Verification items for the finished model (mm, model axes). Coordinates: 2 decimals unless noted, no trailing zeros. Loops run counter-clockwise (first coordinate to the right, second up) from the corner with the lowest first, then second, coordinate; pieces in that order, holes last. Notation, with made-up numbers: (48.25, -34.5) - (84.25, -34.5) arc R20 ccw to (84.25, -26.5) - close; hole circle Ø6 at (-25.75, 26). An arc over 180 degrees is marked (long way). One line per item, written item: value. Start each with the question number.
(1) Section check D-D (x = 24). Record the boundary of the cut face in (y, z), plus the area to 3 significant figures.
(2) Section check A-A (y = 4.5). Record the boundary of the cut face in (x, z).
(3) Thickness scan on probe 1 along Y at (x, z) = (34.5, 2.35); probe 2 along Y at (x, z) = (-5, 4.2); probe 3 along X at (y, z) = (-11.5, 4.1). Record the ranges inside material, lowest first. Write a range as [from, to].
(4) Gauge pin test, flat ends, axial feed: P1, Ø3, axis at y = 7, z = 2.5, coming from the +X side; P2, Ø2, axis at y = 21.5, z = 1, coming from the +X side. Record the tip position at first contact, or that the pin passes through.
(5) Section check B-B (x = 34.5). Record the boundary of the cut face in (y, z).
(6) Section check C-C (z = 3.35). Count the separate pieces of the cut face and the enclosed holes in it, plus the area to 3 significant figures.
Autodesk Inventor part; units mm, degrees
ref_plane "YZ Plane" through (0, 0, 0) normal (1, 0, 0) x (0, 1, 0)
ref_plane "XZ Plane" through (0, 0, 0) normal (0, 1, 0) x (-1, 0, 0)
ref_plane "XY Plane" through (0, 0, 0) normal (0, 0, 1) x (1, 0, 0)
sketch "Base" plane through (0, 0, 0) normal (0, 0, 1) x (1, 0, 0)
  circle A0 centre (14.2875, 0) radius 14.2875 construction
  circle A1 centre (34.9097, 11.9062) radius 1.9939 construction
  circle A2 centre (34.9097, -11.9063) radius 1.9939 construction
  circle A3 centre (14.2875, -23.8125) radius 1.9939 construction
  circle A4 centre (-6.3347, -11.9062) radius 1.9939 construction
  circle A5 centre (-6.3347, 11.9063) radius 1.9939 construction
  circle A6 centre (14.2875, 23.8125) radius 1.9939 construction
  circle A7 centre (14.2875, 0) radius 27.5127
  arc A8 (34.1709, -15.825) -> (37.934, -9.307) centre (34.9097, -11.9063) ccw construction
  circle A9 centre (-6.3347, 11.9063) radius 1.7272
  circle A10 centre (14.2875, 23.8125) radius 1.7272
  circle A11 centre (34.9097, 11.9062) radius 1.7272
  circle A12 centre (34.9097, -11.9063) radius 1.7272
  circle A13 centre (14.2875, -23.8125) radius 1.7272
  circle A14 centre (-6.3347, -11.9062) radius 1.7272
  point P0 (0, 0)
  dimension "d3" = 55.0254
  dimension "d10" = 3.4544
extrude "Plate1" add sketch "Base" along normal blind 5
sketch "WheelMagnetAlignmentFlangeMountHoles" plane through (14.2875, 0, 0) normal (0, 0, -1) x (-1, 0, 0)
  circle A0 centre (4.5, 4.5) radius 1.225
  circle A1 centre (4.5, -4.5) radius 1.225
  circle A2 centre (-4.5, -4.5) radius 1.225
  circle A3 centre (-4.5, 4.5) radius 1.225
  point P0 (14.2875, 0)
extrude "Cut1" cut sketch "WheelMagnetAlignmentFlangeMountHoles" against normal blind 5
equation "\"d45\" = Thickness"
equation "\"d44\" = Thickness"
equation "\"BendRadius\" = Thickness"
equation "\"BendReliefWidth\" = Thickness"
equation "\"BendReliefDepth\" = 0.5 * Thickness"
equation "\"TransitionRadius\" = BendRadius"
equation "\"JacobiRadiusSize\" = BendRadius"
equation "\"GapSize\" = Thickness"
properties part number "LegEncoderHub"
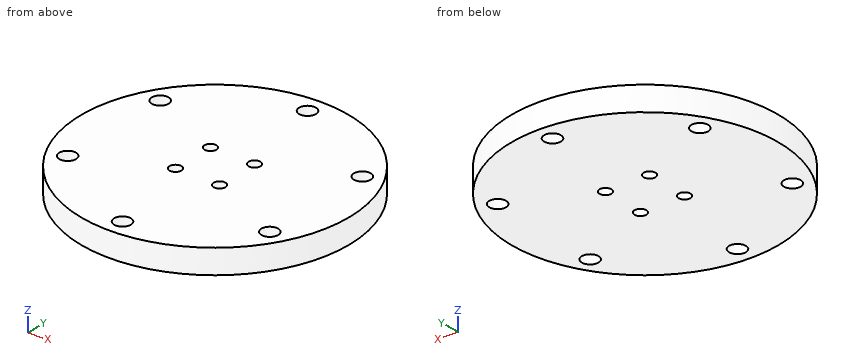
Responses:
1. outline: (-25.74, 0) - (25.74, 0) - (25.74, 5) - (-25.74, 5) - close
1. area: 257 mm²
2. outline: (-12.85, 0) - (8.56, 0) - (8.56, 5) - (-12.85, 5) - close; (11.01, 0) - (17.56, 0) - (17.56, 5) - (11.01, 5) - close; (20.01, 0) - (41.43, 0) - (41.43, 5) - (20.01, 5) - close
3. probe 1: y = [-18.67, -13.58], [-10.23, 10.23], [13.58, 18.67]
3. probe 2: y = [-19.62, -13], [-10.81, 10.81], [13, 19.62]
3. probe 3: x = [-10.71, -8.01], [-4.66, 33.23], [36.59, 39.28]
4. P1: stops at x = 41.24
4. P2: stops at x = 32.64
5. outline: (-18.67, 0) - (-13.58, 0) - (-13.58, 5) - (-18.67, 5) - close; (-10.23, 0) - (10.23, 0) - (10.23, 5) - (-10.23, 5) - close; (13.58, 0) - (18.67, 0) - (18.67, 5) - (13.58, 5) - close
6. separate pieces: 1
6. enclosed holes: 10
6. area: 2,300 mm²
